from build123d import *

# Parameters (mm, degrees)
F0_W     = 253
F0_H     = 254
F1_DEPTH = 1
F2_W     = 253
F2_H     = 254
F2_W_2   = 251
F2_H_2   = 252
F3_DEPTH = 8
F4_W     = 80
F4_H     = 80
F5_DEPTH = 4.2


with BuildPart() as f1:
    # F0 (on Front) → F1 (new body)
    with BuildSketch(Plane.XZ):
        Rectangle(F0_W, F0_H)
    extrude(amount=F1_DEPTH)

    # F2 (on face) → F3 (join)
    with BuildSketch(Plane.XZ.offset(1)):
        Rectangle(F2_W, F2_H)
        Rectangle(F2_W_2, F2_H_2, mode=Mode.SUBTRACT)
    extrude(amount=F3_DEPTH)

    # F4 (on face) → F5 (join)
    with BuildSketch(Plane.XZ.offset(1)):
        Rectangle(F4_W, F4_H)
    extrude(amount=F5_DEPTH)


solid = f1.part
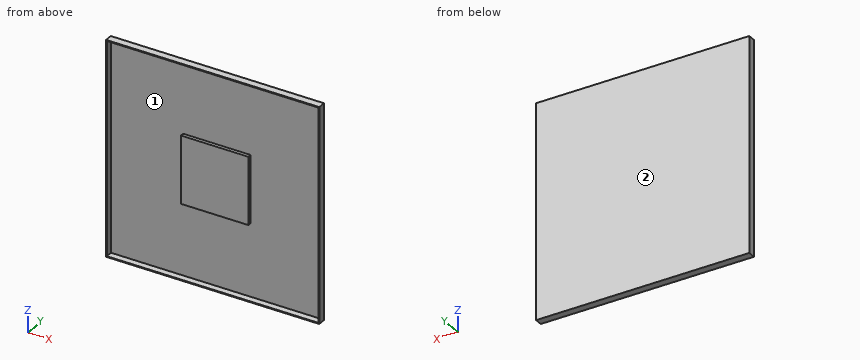
Input: part model. Units: mm. Frame: model coordinates. Face numbers are marked on the shaded views. Coordinates: 2 decimals unless noted, no trailing zeros. Loops run counter-clockwise (first coordinate to the right, second up) from the corner with the lowest first, then second, coordinate; pieces in that order, holes last. Notation, with made-up numbers: (-4, 6.5) -> (11, 6.5) arc R26 cw to (11, 21.5) -> close; hole circle Ø3 at (41, -29.75). An arc over 180 degrees is marked (long way). One line per item, written item: value.
(1) Cut plane D-D (x = -26). Output: boundary loops of the cut face in (y, z).
Answer below:
outline: (-9, -127) -> (0, -127) -> (0, 127) -> (-9, 127) -> (-9, 126) -> (-1, 126) -> (-1, 40) -> (-5.2, 40) -> (-5.2, -40) -> (-1, -40) -> (-1, -126) -> (-9, -126) -> close
(2) Ray query, line 1 along X through (y, z) = (-4.5, 1); line 2 along Z through (x, y) = (-4.5, -3.75); line 3 along Z through (x, y) = (40.5, -2). Return the intervals inside material, ascending.
Answer below:
line 1: x = -126.5 to -125.5, -40 to 40, 125.5 to 126.5
line 2: z = -127 to -126, -40 to 40, 126 to 127
line 3: z = -127 to -126, 126 to 127
(3) Cut plane C-C (z = -31). Output: boundary loops of the cut face in (x, y), then the cut area to 3 significant figures.
Answer below:
outline: (-126.5, -9) -> (-125.5, -9) -> (-125.5, -1) -> (-40, -1) -> (-40, -5.2) -> (40, -5.2) -> (40, -1) -> (125.5, -1) -> (125.5, -9) -> (126.5, -9) -> (126.5, 0) -> (-126.5, 0) -> close
area: 605 mm2
(4) Pin query (flat end, axial travel): pin 1 Ø10 at (x, z) = (-1.5, 31) entering from -Y; pin 2 Ø4 at (x, z) = (70, 66.5) entering from -Y. Return the tip coordinate at first contact, or that it passes through.
Answer below:
pin 1: stops at y = -5.2
pin 2: stops at y = -1
(5) Cut plane A-A (x = 66.5). Output: boundary loops of the cut face in (y, z).
Answer below:
outline: (-9, -127) -> (0, -127) -> (0, 127) -> (-9, 127) -> (-9, 126) -> (-1, 126) -> (-1, -126) -> (-9, -126) -> close
(6) Cut plane B-B (z = -84.5). Output: boundary loops of the cut face in (x, y), then the cut area to 3 significant figures.
Answer below:
outline: (-126.5, -9) -> (-125.5, -9) -> (-125.5, -1) -> (125.5, -1) -> (125.5, -9) -> (126.5, -9) -> (126.5, 0) -> (-126.5, 0) -> close
area: 269 mm2
(7) Draft query along X for the marked faces 1 and 2. Return one class per face: pulls with the +X half, pulls with the -X half, needs draft (parallel to the pull), parting line crosses it, or undercut.
Answer below:
face 1: undercut
face 2: needs draft
